Answer from the drawing. Dimensions are ordinates in mm from the lowest x, y and z of the part. A direction names the side the tool comes from. Coordinates: 2 decimals unless noted, no trailing zeros. Write each loop counter-clockwise with the first axis right and the second up, starting at its lowest first coordinate (ties: lowest second). Pieces come first, ordered by that corner, then holes. Notation, with made-up numbers: (-9, 66.5) -> (5, 66.5) arc R9 cw to (5, 78.5) -> close; hole circle Ø11 at (42.5, 41.25). An arc over 180 degrees is marked (long way). Answer as a JSON object with one key per item and string values. Group by question number.
(1) Flat-ended cylindrical pins translate along their axes: P1, Ø15, axis at x = 28.5, z = 20.5, coming from the +Y side; P2, Ø2, axis at x = 25.5, y = 14, coming from the -Z side; P3, Ø1.5, axis at x = 29.5, y = 13, coming from the +Z side; P4, Ø3.5, axis at x = 26.5, y = 14, coming from the +Z side. Find the tip coordinate at first contact, or state that the pin passes through.
(2) Straight lines are drawn through the part: L1, parallel to Y at x = 2, z = 19; L2, parallel to Z at x = 23, y = 8; L3, parallel to X at y = 9, z = 29. For each, find the intervals that lie inside material, in ascending order.
(3) Which of the six approach directions +Z, -Z, +X, -X, +Y, -Y give full straight-line access (tool end or side, diameter ignored) to the marked faces 4 and 5?
(4) For a pull along Z with two mould halves and no side action, classify the marked faces 1, 2 and 3 as +Z half, -Z half, draft (parallel to the pull), parting line (faces both ways), or undercut.
(5) Find section A-A (y = 10.75). Give the vertices of the cut face in (x, z) (1 decimal).
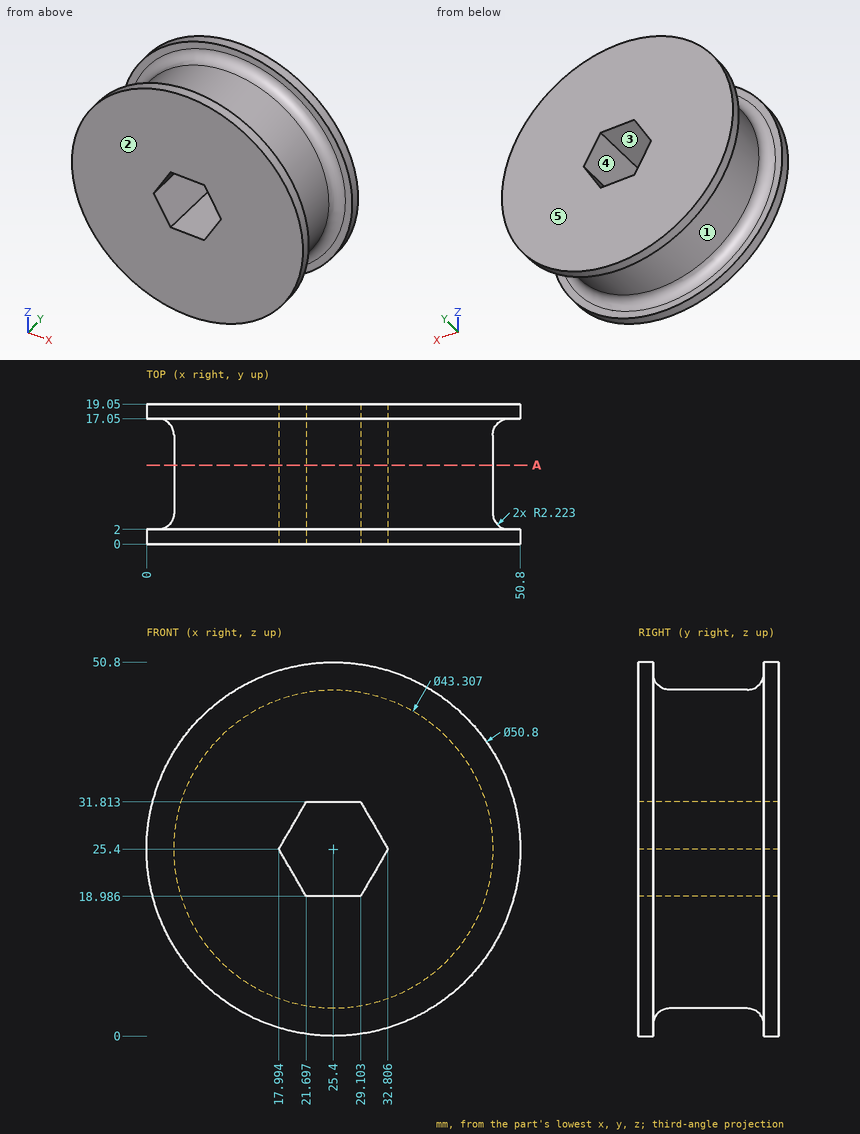
Results below:
{
 "1": {"P1": "stops at y = 19.05", "P2": "stops at z = 3.74", "P3": "stops at z = 46.79", "P4": "stops at z = 47.23"},
 "2": {"L1": "y = 0 to 2, 17.05 to 19.05", "L2": "z = 3.88 to 18.99, 31.81 to 46.92", "L3": "x = 4.05 to 20.07, 30.73 to 46.75"},
 "3": {"face 4": "+Y, -Y", "face 5": "+Z, -Z, +X, -X, +Y"},
 "4": {"face 1": "parting line", "face 2": "draft", "face 3": "undercut"},
 "5": {"outline": "circle Ø43.3 at (25.4, 25.4); hole (18, 25.4) -> (21.7, 19) -> (29.1, 19) -> (32.8, 25.4) -> (29.1, 31.8) -> (21.7, 31.8) -> close"}
}
